CAD build for the part. Positions are in the model's coordinates, mm. A direction names the side the tool comes from. Round coordinates to 2 decimals unless told otherwise and drop trailing zeros. Loops run counter-clockwise (first coordinate to the right, second up) from the corner with the lowest first, then second, coordinate; pieces in that order, holes last. Notation, with made-up numbers: M 11,-8.75 L 53,-8.75 A19 ccw 53,0.25 Z; hole C 54,50 d6. An arc over 180 degrees is marked long. One line per item, written item: value. Start each with the question number.
Autodesk Inventor part; units mm, degrees
ref_plane "YZ Plane" through (0, 0, 0) normal (1, 0, 0) x (0, 1, 0)
ref_plane "XZ Plane" through (0, 0, 0) normal (0, 1, 0) x (-1, 0, 0)
ref_plane "XY Plane" through (0, 0, 0) normal (0, 0, 1) x (1, 0, 0)
sketch "Sketch1" plane through (0, 0, 0) normal (0, 0, 1) x (1, 0, 0)
  circle A0 centre (0, 0) radius 2.5
  line L0 (1.3379, -2.1119) -> (1.34, -2.1119)
  point P0 (-1.3379, -2.1119)
  dimension "d0" = 5
extrude "Extrusion1" add sketch "Sketch1" along normal blind 80
sketch "Sketch2" plane through (0, 0, 0) normal (0, 0, -1) x (-1, 0, 0)
  circle A0 centre (0, 0) radius 2.5
  line L0 (0, -4.6188) -> (-4, -2.3094)
  line L1 (-4, -2.3094) -> (-4, 2.3094)
  line L2 (-4, 2.3094) -> (0, 4.6188)
  line L3 (0, 4.6188) -> (4, 2.3094)
  line L4 (4, 2.3094) -> (4, -2.3094)
  line L5 (4, -2.3094) -> (0, -4.6188)
  dimension "d4" = 8
extrude "Extrusion2" add sketch "Sketch2" against normal blind 4
properties part number "quarter-inch-rod" material "Iron, Cast"
(1) Slice it at A-A, the plane y = -1.5. List the corners of the cut face in (x, z).
(2) Slice it at C-C, the plane x = 0.75. List the corners of the cut face in (y, z).
(3) Probe L1, parallel to Z at x = 0.75, y = -3; L2, parallel to X at y = 0.25, z = 55. List the from-to ranges inside material, lowest first.
(4) Slice it at B-B, the plane z = 61.5. List the corners of the cut face in (x, y).
(5) Flat gauge pin, fed straight in: P1, Ø1.5, axis at x = -2.5, z = 70, coming from the -Y side. Where does the tip first touch, or does it go through?
(6) Which spindle directions (+Z, -Z, +X, -X, +Y, -Y) get a long thin tool onto all of the face, cutting with end or side? Do faces 1 (the flat face through (2.028, 3.448, 1.972)), 2 (the flat face through (-2, -2, 4)). Say none if no direction does.
Check result:
1. outline: M -4,0 L 4,0 L 4,4 L 2,4 L 2,80 L -2,80 L -2,4 L -4,4 Z
2. outline: M -4.19,0 L 4.19,0 L 4.19,4 L 2.38,4 L 2.38,80 L -2.38,80 L -2.38,4 L -4.19,4 Z
3. L1: z = 0 to 4
3. L2: x = -2.49 to 2.49
4. outline: C 0,0 d5
5. P1: stops at y = -1.79
6. face 1: +Z, -Z, +X, +Y
6. face 2: +Z
